```python
from build123d import *

# Parameters (mm, degrees)
BOSS_EXTRUDE1_DEPTH = 3
SKETCH2_R           = 4.7625
BOSS_EXTRUDE2_DEPTH = 5
BOSS_EXTRUDE3_DEPTH = 3
SKETCH4_R           = 2.75
CUT_EXTRUDE1_DEPTH  = 3.5
SKETCH5_R           = 1.25
CUT_EXTRUDE2_DEPTH  = 25.984995497
SKETCH6_R           = 1.75
CUT_EXTRUDE3_DEPTH  = 25.667792767
SKETCH7_R           = 3
CUT_EXTRUDE4_DEPTH  = 2.5


with BuildPart() as part:
    # Sketch1 → Boss-Extrude1 (new body)
    with BuildSketch(Plane(origin=(0, 0, 0), x_dir=(1, 0, 0), z_dir=(0, 1, 0))):
        with BuildLine():
            Line((0, 6), (17.5, 6))
            ThreePointArc((17.5, 6), (23.5, 0), (17.5, -6))
            Line((17.5, -6), (0, -6))
            ThreePointArc((0, -6), (-6, 0), (0, 6))
        make_face()
    extrude(amount=BOSS_EXTRUDE1_DEPTH)

    # Sketch2 → Boss-Extrude2 (add)
    with BuildSketch(Plane(origin=(0, 3, 0), x_dir=(1, 0, 0), z_dir=(0, 1, 0))):
        with Locations(Location((0, 0, 0), (0, 0, 270))):
            Circle(SKETCH2_R)
    extrude(amount=BOSS_EXTRUDE2_DEPTH)

    # Sketch3 → Boss-Extrude3 (add)
    with BuildSketch(Plane(origin=(0, 3, 0), x_dir=(1, 0, 0), z_dir=(0, 1, 0))):
        with BuildLine():
            Line((19.375, -2.875), (14.625, -2.875))
            ThreePointArc((14.625, -2.875), (11.75, 0), (14.625, 2.875))
            Line((14.625, 2.875), (19.375, 2.875))
            ThreePointArc((19.375, 2.875), (22.25, 0), (19.375, -2.875))
        make_face()
    extrude(amount=BOSS_EXTRUDE3_DEPTH)

    # Sketch4 → Cut-Extrude1 (cut)
    with BuildSketch(Plane(origin=(0, 8, 0), x_dir=(1, 0, 0), z_dir=(0, 1, 0))):
        with Locations(Location((0, 0, 0), (0, 0, 270))):
            Circle(SKETCH4_R)
    extrude(amount=-CUT_EXTRUDE1_DEPTH, mode=Mode.SUBTRACT)

    # Sketch5 → Cut-Extrude2 (cut, through all)
    with BuildSketch(Plane(origin=(0, 6, 0), x_dir=(1, 0, 0), z_dir=(0, 1, 0))):
        with Locations(Location((20, 0, 0), (0, 0, 270))):
            Circle(SKETCH5_R)
        with Locations(Location((15, 0, 0), (0, 0, 270))):
            Circle(SKETCH5_R)
    extrude(amount=-CUT_EXTRUDE2_DEPTH, mode=Mode.SUBTRACT)

    # Sketch6 → Cut-Extrude3 (cut, through all)
    with BuildSketch(Plane(origin=(0, 4.5, 0), x_dir=(1, 0, 0), z_dir=(0, 1, 0))):
        with Locations(Location((0, 0, 0), (0, 0, 270))):
            Circle(SKETCH6_R)
    extrude(amount=-CUT_EXTRUDE3_DEPTH, mode=Mode.SUBTRACT)

    # Sketch7 → Cut-Extrude4 (cut)
    with BuildSketch(Plane.XZ):
        with Locations(Location((0, 0, 0), (0, 0, 270))):
            Circle(SKETCH7_R)
    extrude(amount=-CUT_EXTRUDE4_DEPTH, mode=Mode.SUBTRACT)


solid = part.part
```
For this review, take the finished solid that the model builds, in its own axes (mm). A direction names the side the tool comes from. Coordinates: 2 decimals unless noted, no trailing zeros. Order: outer loops, then holes, each group sorted by start corner. A loop starts at its lowest first (then second) coordinate and runs counter-clockwise, first axis right, second up. Notation, with made-up numbers: (-17.5, 80.25) -> (27.5, 80.25) arc R19 ccw to (27.5, 94.25) -> close; hole circle Ø8 at (88, 28.5). An arc over 180 degrees is marked (long way). Answer as CSV lines item,"result".
Q1. We need section D-D (y = 1.5). State the section outline as (x, z) points, plus the area to 3 significant figures.
Model answer:
outline,"(0, -6) -> (17.5, -6) arc R6 ccw to (17.5, 6) -> (0, 6) arc R6 ccw to start; hole circle Ø6 at (0, 0); hole circle Ø2.5 at (15, 0); hole circle Ø2.5 at (20, 0)"
area,"285 mm2"
Q2. For faces 1 (the face through (17, 6, 0)), 2 (the face through (17, 4, 2.875)), 3 (the face through (0.9, 1.23, -2.86)), 4 (the face through (-2.9, 5.46, -3.78)), list the 3-axis set-ups (+Z, -Z, +X, -X, +Y, -Y) from which the entire face can be reached by the end or side of a thin tool; tool diameter is ignored.
Model answer:
face 1,"+Z, -Z, +X, +Y"
face 2,"+Z, +X, +Y"
face 3,"-Y"
face 4,"+Y"
Q3. Wall thickness on line 1 along X through (y, z) = (3.15, 0); line 2 along X through (y, z) = (2.05, 0); line 3 along X through (y, z) = (2.25, 0.5): over which ranges is each line inside the solid? List them lowest first. Write a range as [from, to].
Model answer:
line 1,"x = [-4.76, -1.75], [1.75, 4.76], [11.75, 13.75], [16.25, 18.75], [21.25, 22.25]"
line 2,"x = [-6, -3], [3, 13.75], [16.25, 18.75], [21.25, 23.5]"
line 3,"x = [-5.98, -2.96], [2.96, 13.85], [16.15, 18.85], [21.15, 23.48]"
Q4. Draft analysis for pull direction X (two halves, no side actions). For faces 5 (the face through (-6, 1, 0)), 6 (the face through (9, 1, -6)), 7 (the face through (-2.685, 6.274, -0.596)), state which applies: released by +X, released by -X, zero draft, split by the parting line, or undercut.
Model answer:
face 5,"released by -X"
face 6,"zero draft"
face 7,"undercut"
Q5. Clearance check with flat-ended pins moving along their axes: pin 1 Ø1.6 at (x, z) = (-0.5, 0) entering from +Y; pin 2 Ø6.5 at (x, z) = (0, 0) entering from +Y; pin 3 Ø4.5 at (x, z) = (0, 0) entering from +Y; pin 4 Ø3 at (x, z) = (15, 0) entering from +Y. State where each tip first meets the part, or that it passes through.
Model answer:
pin 1,"passes through"
pin 2,"stops at y = 8"
pin 3,"stops at y = 4.5"
pin 4,"stops at y = 6"
Q6. We need section A-A (x = 15). State the section outline as (y, z) points (3 decimals).
Model answer:
outline,"(0, -6) -> (3, -6) -> (3, -2.875) -> (6, -2.875) -> (6, -1.25) -> (0, -1.25) -> close; (0, 1.25) -> (6, 1.25) -> (6, 2.875) -> (3, 2.875) -> (3, 6) -> (0, 6) -> close"
Q7. We need section B-B (y = 5). Count the separate pieces of the cut face and the enclosed holes in it, plus the area to 3 significant figures.
Model answer:
separate pieces,"2"
enclosed holes,"3"
area,"91.0 mm2"
